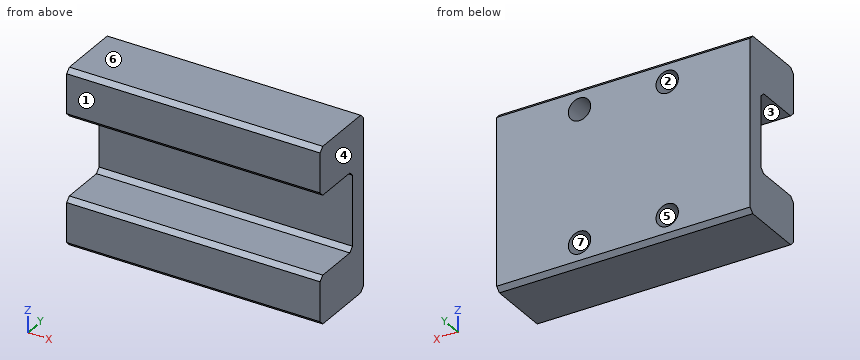
```python
from build123d import *

# Parameters (mm, degrees)
EXTRUDE_1_DEPTH     = 28.9
CHAMFER_1_SIZE      = 0.5
SKETCH_3_R          = 1.275
CUT_EXTRUDE_2_DEPTH = 3


with BuildPart() as part:
    # 草图2 → 拉伸1 (new body)
    with BuildSketch(Plane(origin=(0, 0, 0), x_dir=(0, 0, -1), z_dir=(1, 0, 0))):
        Polygon((-4.5, 0), (4.5, 0), (4.5, -6), (10, -6), (10, 2), (-10, 2), (-10, -6), (-4.5, -6), align=None)
    extrude(amount=EXTRUDE_1_DEPTH)

    # 倒角1
    chamfer_1_edges = [part.edges().sort_by_distance(p)[0] for p in [
        (14.45, -6, 10),
        (14.45, 2, 10),
        (14.45, 2, -10),
        (14.45, -6, -10),
        (14.45, -6, -4.5),
        (14.45, 0, -4.5),
        (14.45, 0, 4.5),
        (14.45, -6, 4.5),
    ]]
    chamfer(chamfer_1_edges, length=CHAMFER_1_SIZE)

    # 草图3 → 拉伸2 (cut)
    with BuildSketch(Plane(origin=(0, 2, 0), x_dir=(1, 0, 0), z_dir=(0, 1, 0))):
        with Locations(Location((9.45, 7.5, 0), (0, 0, 270))):
            Circle(SKETCH_3_R)
        with Locations(Location((19.45, 7.5, 0), (0, 0, 90))):
            Circle(SKETCH_3_R)
        with Locations(Location((19.45, -7.5, 0), (0, 0, 270))):
            Circle(SKETCH_3_R)
        with Locations(Location((9.45, -7.5, 0), (0, 0, 90))):
            Circle(SKETCH_3_R)
    extrude(amount=-CUT_EXTRUDE_2_DEPTH, mode=Mode.SUBTRACT)


solid = part.part
```
The model under review builds one solid part; all positions refer to its coordinate system, in mm. Face numbers are marked on the shaded views. A direction names the side the tool comes from. Round coordinates to 2 decimals unless told otherwise and drop trailing zeros. Write each loop counter-clockwise with the first axis right and the second up, starting at its lowest first coordinate (ties: lowest second). Pieces come first, ordered by that corner, then holes. Notation, with made-up numbers: (83, 41.25) - (126, 41.25) arc R32 cw to (126, 68.25) - close; hole circle Ø2 at (31, -12). An arc over 180 degrees is marked (long way). Answer as CSV lines item,"result". Start each with the question number.
(1) We need section D-D on z = 7.5. State the section outline as (x, y) points (3 decimals), plus the area to 3 significant figures.
(2) To check wall thickness, follow line 1 (X direction, y = 1.1, z = 7.5) (3 decimals); line 2 (Z direction, x = 14.25, y = -2.5); line 3 (X direction, y = -0.25, z = -7). State the ranges of each line that lie inside material, in increasing order.
(3) For pin 1 Ø1.3 at (x, z) = (9.5, -8) entering from +Y, flat-tipped, find the tip position at first contact; note if it passes through.
(4) We need section B-B on x = 19.45. State the section outline as (y, z) points (3 decimals), plus the area to 3 significant figures.
(5) Draft analysis for pull direction X (two halves, no side actions). For the marked faces 4, 5, 6 and 7, state which applies: pulls with the +X half, pulls with the -X half, needs draft (parallel to the pull), parting line crosses it, or undercut.
(6) For the marked faces 1, 2 and 3, list the 3-axis set-ups (+Z, -Z, +X, -X, +Y, -Y) from which the entire face can be reached by the end or side of a thin tool; tool diameter is ignored.
(7) We need section A-A on y = -2.5. State the section outline as (x, z) points.
(8) We need section C-C on y = 1. State the section outline as (x, z) points (3 decimals), plus the area to 3 significant figures.
Worked answers:
1,outline,"(0, -6) - (28.9, -6) - (28.9, 2) - (20.725, 2) - (20.725, -1) - (18.175, -1) - (18.175, 2) - (10.725, 2) - (10.725, -1) - (8.175, -1) - (8.175, 2) - (0, 2) - close"
1,area,"216 mm²"
2,line 1,"0 to 8.175, 10.725 to 18.175, 20.725 to 28.9"
2,line 2,"-10 to -4.5, 4.5 to 10"
2,line 3,"0 to 8.28, 10.62 to 18.28, 20.62 to 28.9"
3,pin 1,"y = -1"
4,outline,"(-6, -9.5) - (-5.5, -10) - (1.5, -10) - (2, -9.5) - (2, -8.775) - (-1, -8.775) - (-1, -6.225) - (2, -6.225) - (2, 6.225) - (-1, 6.225) - (-1, 8.775) - (2, 8.775) - (2, 9.5) - (1.5, 10) - (-5.5, 10) - (-6, 9.5) - (-6, 5) - (-5.5, 4.5) - (-0.5, 4.5) - (0, 4) - (0, -4) - (-0.5, -4.5) - (-5.5, -4.5) - (-6, -5) - close"
4,area,"90.2 mm²"
5,face 4,"pulls with the +X half"
5,face 5,"undercut"
5,face 6,"needs draft"
5,face 7,"undercut"
6,face 1,"+Z, -Z, +X, -X, -Y"
6,face 2,"+Y"
6,face 3,"+X, -X, -Y"
7,outline,"(0, -10) - (28.9, -10) - (28.9, -4.5) - (0, -4.5) - close; (0, 4.5) - (28.9, 4.5) - (28.9, 10) - (0, 10) - close"
8,outline,"(0, -10) - (28.9, -10) - (28.9, 10) - (0, 10) - close; hole circle Ø2.55 at (9.45, -7.5); hole circle Ø2.55 at (9.45, 7.5); hole circle Ø2.55 at (19.45, -7.5); hole circle Ø2.55 at (19.45, 7.5)"
8,area,"558 mm²"
